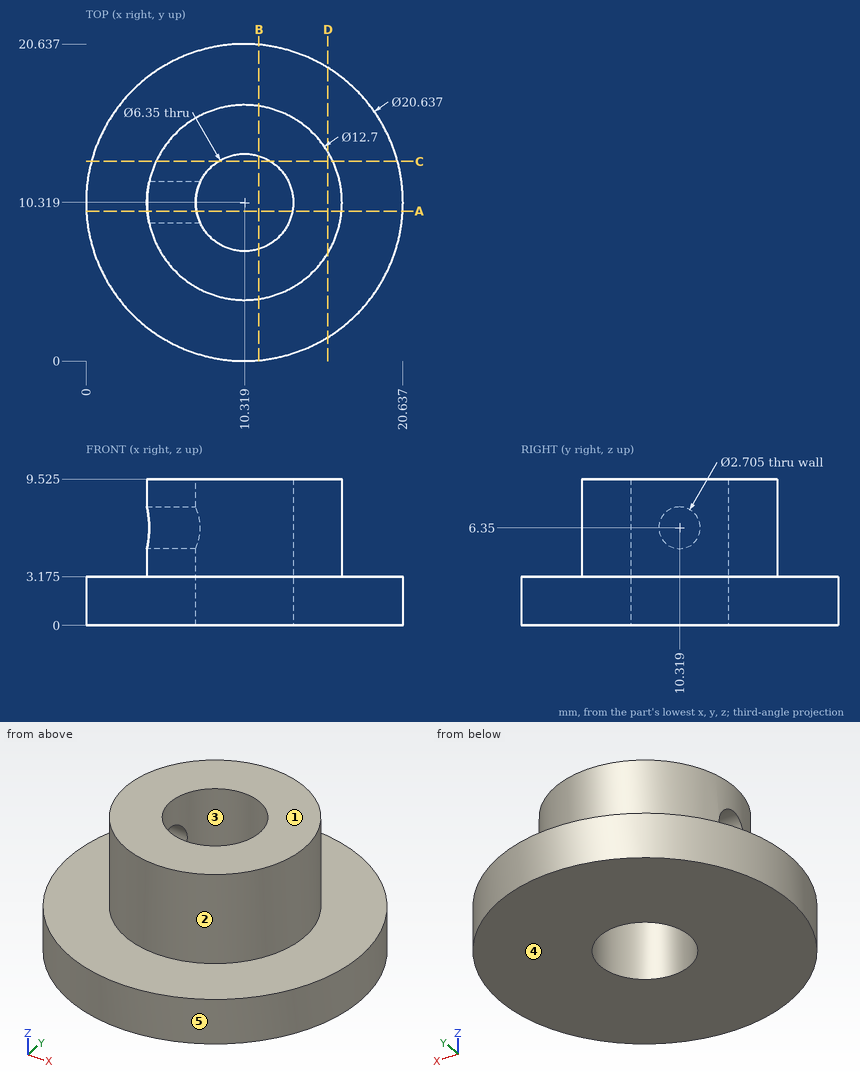
Study the drawing (mm; zero at the part's minimum x, y, z) and answer. A direction names the side the tool comes from. Give positions to 0.01 mm unless a question says otherwise; leave off trailing zeros. Loops run counter-clockwise (first coordinate to the right, second up) from the corner with the lowest first, then second, coordinate; pieces in that order, holes last. Notation, with made-up numbers: M 47,-25.5 L 62,-25.5 A11 cw 62,-7.5 Z; hole C 16,-2.75 d5. An arc over 180 degrees is marked long. Answer as CSV lines item,"result".
Item 1: The part is cut by section C-C (y = 13). Give the vertices of the cut face in (x, z) (1 decimal), and give its area (3 significant figures).
Values follow:
outline,"M 0.4,0 L 8.6,0 L 8.6,9.5 L 4.6,9.5 L 4.6,3.2 L 0.4,3.2 Z; M 12,0 L 20.3,0 L 20.3,3.2 L 16.1,3.2 L 16.1,9.5 L 12,9.5 Z"
area,"104 mm^2"
Item 2: The part is cut by section B-B (x = 11.25). Give the vertices of the cut face in (y, z) (1 decimal).
Values follow:
outline,"M 0,0 L 7.3,0 L 7.3,9.5 L 4,9.5 L 4,3.2 L 0,3.2 Z; M 13.4,0 L 20.6,0 L 20.6,3.2 L 16.6,3.2 L 16.6,9.5 L 13.4,9.5 Z"
Item 3: Given pin 1 Ø1 at (y, z) = (16.5, 2.5) entering from -X (1 decimal); pin 2 Ø5 at (y, z) = (2.5, 1.5) entering from +X; pin 3 Ø3.5 at (y, z) = (10.32, 6.35) entering from +X, each flat-ended and moving along its own axis, determine where each tip first touches the part or whether it passes through.
Values follow:
pin 1,"stops at x = 1.7"
pin 2,"stops at x = 19.16"
pin 3,"stops at x = 16.67"
Item 4: The part is cut by section D-D (x = 15.75). Give the vertices of the cut face in (y, z) (1 decimal).
Values follow:
outline,"M 1.5,0 L 19.1,0 L 19.1,3.2 L 13.6,3.2 L 13.6,9.5 L 7,9.5 L 7,3.2 L 1.5,3.2 Z"
Item 5: The mould has two halves that part along Y. Classify the marked faces 3, 4 and 5: released by +Y, released by -Y, zero draft, split by the parting line, or undercut.
Values follow:
face 3,"undercut"
face 4,"zero draft"
face 5,"split by the parting line"
Item 6: Straight lines are drawn through the part: line 1 along Y through (x, z) = (5.55, 6.35) (1 decimal); line 2 along Y through (x, z) = (7, 7.25) (1 decimal); line 3 along X through (y, z) = (12.5, 7.5) (1 decimal). For each, find the intervals that lie inside material, in ascending order. Write a range as [from, to].
Values follow:
line 1,"y = [6.1, 9], [11.7, 14.5]"
line 2,"y = [4.9, 9.3], [11.3, 15.7]"
line 3,"x = [4.4, 8], [12.6, 16.3]"
Item 7: Which of the six approach directions +Z, -Z, +X, -X, +Y, -Y give full straight-line access (tool end or side, diameter ignored) to the marked faces 1 and 2?
Values follow:
face 1,"+Z, +X, -X, +Y, -Y"
face 2,"+Z"
Item 8: The part is cut by section A-A (y = 9.75). Give the vertices of the cut face in (x, z) (1 decimal).
Values follow:
outline,"M 0,0 L 7.2,0 L 7.2,5.1 L 4,5.1 L 4,3.2 L 0,3.2 Z; M 4,7.6 L 7.2,7.6 L 7.2,9.5 L 4,9.5 Z; M 13.4,0 L 20.6,0 L 20.6,3.2 L 16.6,3.2 L 16.6,9.5 L 13.4,9.5 Z"
